Design review of the part built by this model. Coordinates are the model's own, in mm. Coordinates: 2 decimals unless noted, no trailing zeros. Write each loop counter-clockwise with the first axis right and the second up, starting at its lowest first coordinate (ties: lowest second). Pieces come first, ordered by that corner, then holes.
Q1. For probe 1 along Z at (x, y) = (41.5, 143.5); probe 2 along Z at (x, y) = (120.5, 144.5); probe 3 along Z at (x, y) = (-70, 41.5) (3 decimals), list the stretches that pass through material, from the lowest coordinate up.
Q2. Insertion check: pin 1 (6 mm diameter, centred on x = -86, y = 112.5, fed in from +Z); pin 2 (20 mm diameter, centred on x = 4.5, z = -3, fed in from -Y); pin 3 (6 mm diameter, centred on x = 90, y = 167, fed in from +Z); pin 4 (10 mm diameter, centred on x = 93, y = 93, fed in from -Z). Each pin has a flat end and moves straight along its axis. Give the tip position at first contact, or say it passes through.
Q3. Take a section at C-C (y = 51). State how many separate pieces and enclosed holes the cut face has, and give its area (3 significant figures).
Q4. Take a section at D-D (x = 17.5). Give the boundary of the cut face in (y, z), and give its area (3 significant figures).
Q5. Mouldability with a two-part tool opening along Z and no side actions: class faces 1 (the cylindrical face through (-91.273, 108.46, -119.035)), 2 (the flat face through (0, 210, 0)), 3 (the flat face through (-31, 0, -2)) as pulls with the +Z half, pulls with the -Z half, needs draft (parallel to the pull), parting line crosses it, or undercut.
Q6. Take a section at B-B (x = -101). Give the boundary of the cut face in (y, z).
Q7. Take a section at A-A (z = -67.5). Give the boundary of the cut face in (x, y), and give its area (3 significant figures).
```python
from build123d import *

# Parameters (mm, degrees)
SKETCH_1_R      = 150
SKETCH_1_R_2    = 36
EXTRUDE_1_DEPTH = 220
EXTRUDE_START   = -10
SKETCH_2_R      = 12.5
EXTRUDE_2_DEPTH = 10


with BuildPart() as part:
    # 草圖1 → 填料-伸長1 (new body)
    with BuildSketch(Plane(origin=(0, 0, 0), x_dir=(1, 0, 0), z_dir=(0, 1, 0))):
        with Locations(Location((0, 0, 0), (0, 0, 270))):
            Circle(SKETCH_1_R)
        with Locations(Location((0, 110, 0), (0, 0, 270))):
            Circle(SKETCH_1_R_2, mode=Mode.SUBTRACT)
        with Locations(Location((70.706637066, 84.264888743, 0), (0, 0, 270))):
            Circle(SKETCH_1_R_2, mode=Mode.SUBTRACT)
        with Locations(Location((108.328852831, 19.101299543, 0), (0, 0, 270))):
            Circle(SKETCH_1_R_2, mode=Mode.SUBTRACT)
        with Locations(Location((95.262794416, -55, 0), (0, 0, 270))):
            Circle(SKETCH_1_R_2, mode=Mode.SUBTRACT)
        with Locations(Location((37.622215766, -103.366188286, 0), (0, 0, 270))):
            Circle(SKETCH_1_R_2, mode=Mode.SUBTRACT)
        with Locations(Location((-37.622215766, -103.366188286, 0), (0, 0, 270))):
            Circle(SKETCH_1_R_2, mode=Mode.SUBTRACT)
        with Locations(Location((-95.262794416, -55, 0), (0, 0, 270))):
            Circle(SKETCH_1_R_2, mode=Mode.SUBTRACT)
        with Locations(Location((-108.328852831, 19.101299543, 0), (0, 0, 270))):
            Circle(SKETCH_1_R_2, mode=Mode.SUBTRACT)
        with Locations(Location((-70.706637066, 84.264888743, 0), (0, 0, 270))):
            Circle(SKETCH_1_R_2, mode=Mode.SUBTRACT)
        with BuildLine():
            ThreePointArc((12.247448714, 2.5), (-12.5, 0), (12.247448714, -2.5))
            ThreePointArc((12.247448714, -2.5), (12.5, 0), (12.247448714, 2.5))
        make_face(mode=Mode.SUBTRACT)
    extrude(amount=EXTRUDE_1_DEPTH)

    # 草圖2 → 填料-伸長2 (add)
    with BuildSketch(Plane(origin=(0, 220, 0), x_dir=(1, 0, 0), z_dir=(0, 1, 0)).offset(EXTRUDE_START)):
        with Locations(Location((0, 0, 0), (0, 0, 270))):
            Circle(SKETCH_2_R)
    extrude(amount=EXTRUDE_2_DEPTH)


solid = part.part
```
Response:
1. probe 1: z = -144.14 to -105.31, -63.22 to 67.58, 139.16 to 144.14
1. probe 2: z = -89.33 to -52.98, 14.78 to 29.33, 80.67 to 89.33
1. probe 3: z = -132.665 to -120.258, -48.272 to 29.353, 80.647 to 87.628, 119.104 to 132.665
2. pin 1: stops at z = 124.94
2. pin 2: stops at y = 0
2. pin 3: stops at z = 122.19
2. pin 4: stops at z = -121.47
3. separate pieces: 1
3. enclosed holes: 10
3. area: 33,600 mm2
4. outline: (0, -148.98) - (220, -148.98) - (220, -141.46) - (0, -141.46) - close; (0, -78.54) - (220, -78.54) - (220, 73.51) - (0, 73.51) - close; (0, 133.22) - (220, 133.22) - (220, 148.98) - (0, 148.98) - close
4. area: 38,600 mm2
5. face 1: parting line crosses it
5. face 2: undercut
5. face 3: needs draft
6. outline: (0, -110.9) - (220, -110.9) - (220, -103.72) - (0, -103.72) - close; (0, -64.81) - (220, -64.81) - (220, -54.35) - (0, -54.35) - close; (0, 16.14) - (220, 16.14) - (220, 19.46) - (0, 19.46) - close; (0, 90.54) - (220, 90.54) - (220, 110.9) - (0, 110.9) - close
7. outline: (-133.95, 0) - (-102.56, 0) - (-102.56, 220) - (-133.95, 220) - close; (-38.85, 0) - (38.85, 0) - (38.85, 220) - (-38.85, 220) - close; (102.56, 0) - (133.95, 0) - (133.95, 220) - (102.56, 220) - close
7. area: 30,900 mm2
